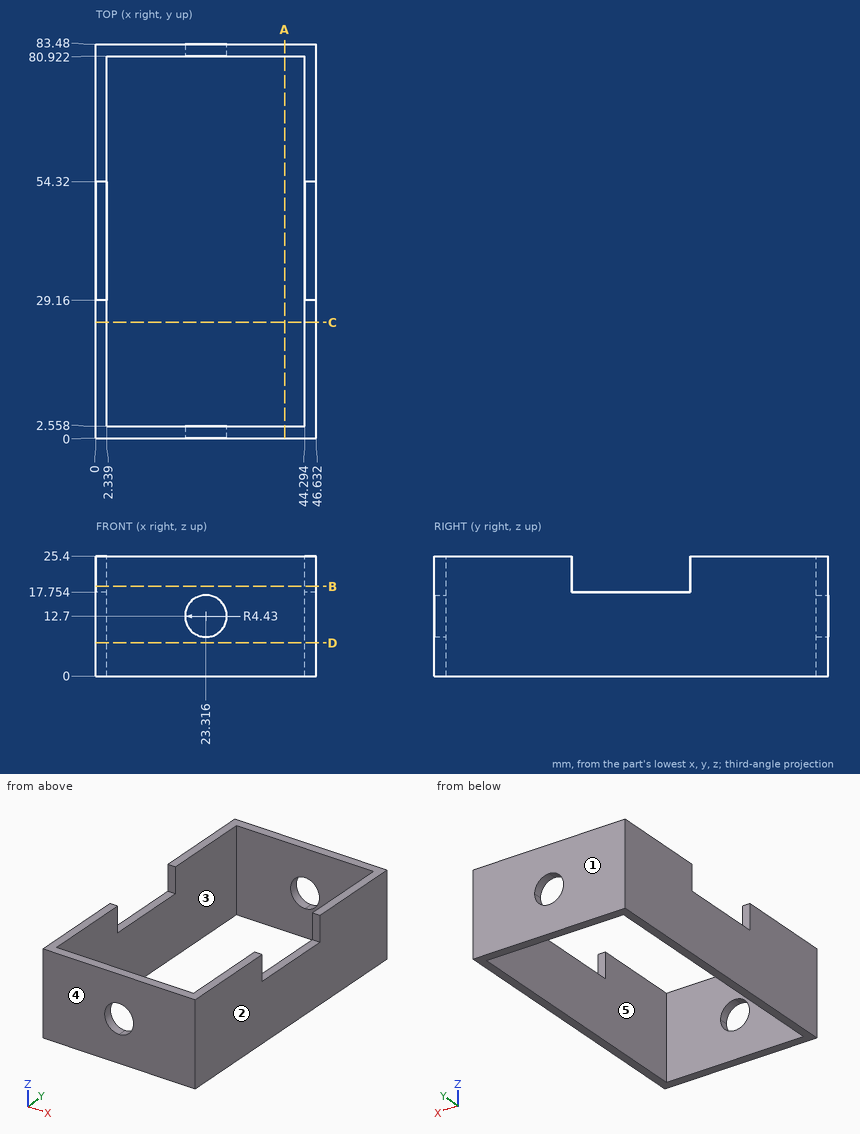
Design review of the part shown in the three views and the two pictorial views. Dimensions are in mm from the part's minimum x, y and z. A direction names the side the tool comes from. Give positions to 0.01 mm unless a question says otherwise; leave off trailing zeros. Write each loop counter-clockwise with the first axis right and the second up, starting at its lowest first coordinate (ties: lowest second). Pieces come first, ordered by that corner, then holes.
(1) Clearance check with a flat-ended pin moving along its axis: pin 1 Ø1.9 at (x, y) = (0.5, 47) entering from +Z. State where the tip first meets the part, or that it passes through.
Checked values:
pin 1: stops at z = 17.75
(2) Wall thickness on line 1 along Y through (x, z) = (33.5, 22); line 2 along X through (y, z) = (72, 16): over which ranges is each line inside the solid? List them lowest first.
Checked values:
line 1: y = 0 to 2.56, 80.92 to 83.48
line 2: x = 0 to 2.34, 44.29 to 46.63
(3) Add section A-A (x = 40). Give the boundary of the cut face in (y, z), and give its area (3 significant figures).
Checked values:
outline: (0, 0) - (2.56, 0) - (2.56, 25.4) - (0, 25.4) - close; (80.92, 0) - (83.48, 0) - (83.48, 25.4) - (80.92, 25.4) - close
area: 130 mm2
(4) Mouldability with a two-part tool opening along Y and no side actions: class the marked faces 1, 2 and 3 as +Y half, -Y half, draft (parallel to the pull), parting line (faces both ways), or undercut.
Checked values:
face 1: +Y half
face 2: draft
face 3: undercut
(5) Add section D-D (z = 7). Give the boundary of the cut face in (x, y).
Checked values:
outline: (0, 0) - (46.63, 0) - (46.63, 83.48) - (0, 83.48) - close; hole (2.34, 2.56) - (44.29, 2.56) - (44.29, 80.92) - (2.34, 80.92) - close
(6) Add section B-B (z = 19). Give the boundary of the cut face in (x, y).
Checked values:
outline: (0, 0) - (46.63, 0) - (46.63, 29.16) - (44.29, 29.16) - (44.29, 2.56) - (2.34, 2.56) - (2.34, 29.16) - (0, 29.16) - close; (0, 54.32) - (2.34, 54.32) - (2.34, 80.92) - (44.29, 80.92) - (44.29, 54.32) - (46.63, 54.32) - (46.63, 83.48) - (0, 83.48) - close
(7) Tool access review of the marked faces 4 and 5: name each direction out of +Z, -Z, +X, -X, +Y, -Y from which nothing blocks a thin tool from reaching the whole face with its end or side.
Checked values:
face 4: +Z, -Z, +X, -X, -Y
face 5: +Z, -Z
(8) Add section C-C (y = 24.5). Give the boundary of the cut face in (x, z), and give its area (3 significant figures).
Checked values:
outline: (0, 0) - (2.34, 0) - (2.34, 25.4) - (0, 25.4) - close; (44.29, 0) - (46.63, 0) - (46.63, 25.4) - (44.29, 25.4) - close
area: 119 mm2
